```python
from build123d import *

# Parameters (mm, degrees)
BOSS_EXTRUDE1_DEPTH = 444.5
SKETCH3_R           = 1.651
SKETCH3_R_2         = 4.826
SKETCH3_R_3         = 1.5875
CUT_EXTRUDE1_DEPTH  = 446.700343561
SKETCH4_R           = 3.175
CUT_EXTRUDE2_DEPTH  = 447.547694121
LPATTERN1_COUNT     = 35
LPATTERN1_PITCH     = 25.4


with BuildPart() as part:
    # Sketch2 → Boss-Extrude1 (new, symmetric)
    with BuildSketch(Plane(origin=(0, 0, 0), x_dir=(1, 0, 0), z_dir=(0, 1, 0))):
        with BuildLine():
            Line((-12.7, 0), (-12.7, 22.225))
            ThreePointArc((-12.7, 22.225), (-11.77006403, 24.47006403), (-9.525, 25.4))
            Line((-9.525, 25.4), (9.525, 25.4))
            ThreePointArc((9.525, 25.4), (11.77006403, 24.47006403), (12.7, 22.225))
            Line((12.7, 22.225), (12.7, 0))
            Line((12.7, 0), (15.875, 0))
            Line((15.875, 0), (15.875, 22.225))
            ThreePointArc((15.875, 22.225), (14.015128061, 26.715128061), (9.525, 28.575))
            Line((9.525, 28.575), (-9.525, 28.575))
            ThreePointArc((-9.525, 28.575), (-14.015128061, 26.715128061), (-15.875, 22.225))
            Line((-15.875, 22.225), (-15.875, 0))
            Line((-15.875, 0), (-12.7, 0))
        make_face()
    extrude(amount=BOSS_EXTRUDE1_DEPTH, both=True)

    # Sketch3 → Cut-Extrude1 (cut, through all)
    with BuildSketch(Plane(origin=(0, 0, -28.575), x_dir=(-1, 0, 0), z_dir=(0, 0, -1))):
        with Locations((0, 444.5)):
            Circle(SKETCH3_R)
        with Locations((-2.032, 361.95)):
            Circle(SKETCH3_R_2)
        with Locations((-2.032, 336.55)):
            Circle(SKETCH3_R_2)
        with Locations((-2.032, 107.95)):
            Circle(SKETCH3_R_2)
        with Locations((-2.032, 82.55)):
            Circle(SKETCH3_R_2)
        with Locations((-2.032, -107.95)):
            Circle(SKETCH3_R_2)
        with Locations((-2.032, -82.55)):
            Circle(SKETCH3_R_2)
        with Locations((0, -241.3)):
            Circle(SKETCH3_R_3)
        with Locations((2.032, 0)):
            Circle(SKETCH3_R_2)
        with Locations((-2.032, -336.55)):
            Circle(SKETCH3_R_2)
        with Locations((-2.032, -361.95)):
            Circle(SKETCH3_R_2)
    extrude(amount=-CUT_EXTRUDE1_DEPTH, mode=Mode.SUBTRACT)

    # Sketch4 → Cut-Extrude2 (cut, through all)
    with BuildSketch(Plane(origin=(15.875, 0, 0), x_dir=(0, 0, -1), z_dir=(1, 0, 0))):
        with Locations((15.875, 431.8)):
            Circle(SKETCH4_R)
    cut_extrude2 = extrude(amount=-CUT_EXTRUDE2_DEPTH, mode=Mode.SUBTRACT)

    # LPattern1: Cut-Extrude2 ×35
    with Locations(*[(0, -i * LPATTERN1_PITCH, 0) for i in range(1, LPATTERN1_COUNT)]):
        add(cut_extrude2, mode=Mode.SUBTRACT)


solid = part.part
```
Geometry check sheet. Reference: the model listing, model coordinates, mm. A direction names the side the tool comes from. Give positions to 0.01 mm unless a question says otherwise; leave off trailing zeros. Write each loop counter-clockwise with the first axis right and the second up, starting at its lowest first coordinate (ties: lowest second). Pieces come first, ordered by that corner, then holes.
1) Material ranges on L1, parallel to X at y = 324, z = -4 (3 decimals); L2, parallel to Z at x = 14.1, y = 304.8; L3, parallel to Z at x = -4, y = -96.5 (3 decimals), recorded low to high.
2) Section check A-A, the plane z = -4.75. Record the boundary of the cut face in (x, y) (3 decimals).
3) Release check for a two-part mould opening along X. For faces 3 (the flat face through (0, 6, -25.4)), 4 (the flat face through (0, 6, -28.575)), 5 (the flat face through (-15.875, 6, -11)), 6 (the flat face through (-12.7, 6, -11)) record: pulls with the +X half, pulls with the -X half, needs draft (parallel to the pull), parting line crosses it, or undercut.
4) Access from +Z, -Z, +X, -X, +Y, -Y to the whole of each face (thin tool, end or side, straight path). Record for faces 1 (the flat face through (12.7, 6, -11)), 2 (the flat face through (0, -444.5, -26)).
5) Gauge pin test, flat ends, axial feed: pin 1 (8 mm diameter, centred on x = -2, y = 22, fed in from +Z); pin 2 (4 mm diameter, centred on x = -8.5, y = -133.5, fed in from +Z). Record the tip position at first contact, or that the pin passes through.
Computed:
1. L1: x = -15.875 to -12.7, 12.7 to 15.875
1. L2: z = -26.63 to -19.05, -12.7 to 0
1. L3: z = -28.575 to -25.4
2. outline: (-15.875, -444.5) - (-12.7, -444.5) - (-12.7, 444.5) - (-15.875, 444.5) - close; (12.7, -444.5) - (15.875, -444.5) - (15.875, 444.5) - (12.7, 444.5) - close
3. face 3: undercut
3. face 4: needs draft
3. face 5: pulls with the -X half
3. face 6: undercut
4. face 1: +Z, +Y, -Y
4. face 2: +Z, -Z, +X, -X, -Y
5. pin 1: stops at z = -25.4
5. pin 2: stops at z = -25.25
